from build123d import *

# Parameters (mm, degrees)
SKETCH_1_R      = 20
EXTRUDE_1_DEPTH = 2
SKETCH_2_W      = 4
SKETCH_2_H      = 4
EXTRUDE_2_DEPTH = 2


with BuildPart() as part:
    # 草图1 → 凸台-拉伸1 (new body)
    with BuildSketch(Plane.XY):
        Circle(SKETCH_1_R)
    extrude(amount=EXTRUDE_1_DEPTH)

    # 草图2 → 凸台-拉伸2 (add)
    with BuildSketch(Plane.XY):
        with Locations((21, 0)):
            Rectangle(SKETCH_2_W, SKETCH_2_H)
        with Locations((0, 21)):
            Rectangle(SKETCH_2_W, SKETCH_2_H)
        with Locations((-21, 0)):
            Rectangle(SKETCH_2_W, SKETCH_2_H)
        with Locations((0, -21)):
            Rectangle(SKETCH_2_W, SKETCH_2_H)
    extrude(amount=EXTRUDE_2_DEPTH)


solid = part.part
The model under review builds one solid part; all positions refer to its coordinate system, in mm. A direction names the side the tool comes from. Give positions to 0.01 mm unless a question says otherwise; leave off trailing zeros. Loops run counter-clockwise (first coordinate to the right, second up) from the corner with the lowest first, then second, coordinate; pieces in that order, holes last. Notation, with made-up numbers: (61, 28.5) -> (98, 28.5) arc R17 cw to (98, 56.5) -> close; hole circle Ø10 at (72.25, 32.5). An arc over 180 degrees is marked (long way). Answer as a JSON object with one key per item and string values. Group by question number.
Q1. Tool access review of faces 1 (the flat face through (-21, 2, 1)), 2 (the flat face through (21, 2, 1)), 3 (the flat face through (-2, -21, 1)), 4 (the flat face through (21, -2, 1)): name each direction out of +Z, -Z, +X, -X, +Y, -Y from which nothing blocks a thin tool from reaching the whole face with its end or side.
Q2. Take a section at B-B (y = -8.5). Write out the cut boundary in (x, z), plus the area to 3 significant figures.
Q3. Insertion check: pin 1 (1 mm diameter, centred on y = 22, z = 1.5, fed in from +X); pin 2 (1 mm diameter, centred on x = 17, z = 1.5, fed in from -Y). Each pin has a flat end and moves straight along its axis. Give the tip position at first contact, or say it passes through.
Q4. Take a section at C-C (x = 3). Write out the cut boundary in (y, z), plus the area to 3 significant figures.
Q5. Take a section at A-A (z = 0.3). Write out the cut boundary in (x, y).
Q6. Wall thickness on line 1 along X through (y, z) = (20.5, 1.25); line 2 along X through (y, z) = (-15.5, 0.6); line 3 along Y through (x, z) = (12.5, 1.25): over which ranges is each line inside the solid? List them lowest first.
Answer below:
{
 "1": {"face 1": "+Z, -Z, -X, +Y", "face 2": "+Z, -Z, +X, +Y", "face 3": "+Z, -Z, -X, -Y", "face 4": "+Z, -Z, +X, -Y"},
 "2": {"outline": "(-18.1, 0) -> (18.1, 0) -> (18.1, 2) -> (-18.1, 2) -> close", "area": "72.4 mm2"},
 "3": {"pin 1": "stops at x = 2", "pin 2": "stops at y = -11.3"},
 "4": {"outline": "(-19.77, 0) -> (19.77, 0) -> (19.77, 2) -> (-19.77, 2) -> close", "area": "79.1 mm2"},
 "5": {"outline": "(-23, -2) -> (-19.9, -2) arc R20 ccw to (-2, -19.9) -> (-2, -23) -> (2, -23) -> (2, -19.9) arc R20 ccw to (19.9, -2) -> (23, -2) -> (23, 2) -> (19.9, 2) arc R20 ccw to (2, 19.9) -> (2, 23) -> (-2, 23) -> (-2, 19.9) arc R20 ccw to (-19.9, 2) -> (-23, 2) -> close"},
 "6": {"line 1": "x = -2 to 2", "line 2": "x = -12.64 to 12.64", "line 3": "y = -15.61 to 15.61"}
}
